Verification items for the finished model (mm, model axes). A direction names the side the tool comes from. Round coordinates to 2 decimals unless told otherwise and drop trailing zeros. Write each loop counter-clockwise with the first axis right and the second up, starting at its lowest first coordinate (ties: lowest second). Pieces come first, ordered by that corner, then holes. Notation, with made-up numbers: (20.5, -14) -> (37.5, -14) arc R17 cw to (37.5, 3) -> close; hole circle Ø11 at (21, 75.25). An arc over 180 degrees is marked (long way). Use CSV: the item, a comma, the result in double quotes.
```python
from build123d import *

# Parameters (mm, degrees)
FILLET1_R = 10


with BuildPart() as part:
    # Sketch1 → Revolve1 (revolve)
    with BuildSketch(Plane.XY, mode=Mode.PRIVATE) as revolve1_sk:
        Polygon((0, 406.66959799), (0, 416.66959799), (-100, 416.66959799), (-195, -406.33040201), (0, -406.33040201), (0, -396.33040201), (-188.812485751, -396.33040201), (-96.121112726, 406.66959799), align=None)
    revolve(revolve1_sk.sketch.rotate(Axis((0, 416.66959799, 0), (0, -1, 0)), 270), axis=Axis((0, 416.66959799, 0), (0, -1, 0)))

    # Fillet1
    fillet1_edges = [part.edges().sort_by_distance(p)[0] for p in [
        (0, 416.66959799, -100),
    ]]
    fillet(fillet1_edges, radius=FILLET1_R)


solid = part.part
```
Q1. Section check C-C (y = 112). Record the cut outline in (x, z), plus the area to 3 significant figures.
Filled in:
outline,"circle Ø270.34 at (0, 0); hole circle Ø260.27 at (0, 0)"
area,"4,200 mm²"
Q2. Section check D-D (y = -38.5). Record the cut outline in (x, z), plus the area to 3 significant figures.
Filled in:
outline,"circle Ø305.08 at (0, 0); hole circle Ø295.02 at (0, 0)"
area,"4,740 mm²"
Q3. Go/stop test with flat-tipped pins: P1, Ø1.5, axis at y = 105, z = 80.5, coming from the +X side; P2, Ø8, axis at y = 277.5, z = -52, coming from the +X side; P3, Ø3, axis at x = -97.5, z = -24, coming from the +Y side. Record where each tip stops, or that it passes through.
Filled in:
P1,"x = 110.14"
P2,"x = 105.74"
P3,"y = 412.9"
Q4. Mould release check, pull along Z, two halves, no side actions. Record for faces 1 (the flat face through (-3, -396.33, 3)), 2 (the flat face through (-1, 416.67, 1)), 3 (the conical face through (-44.656, -4.956, 141.804)): released by +Z, released by -Z, zero draft, split by the parting line, or undercut.
Filled in:
face 1,"undercut"
face 2,"zero draft"
face 3,"split by the parting line"
Q5. Section check A-A (z = 0). Record the cut outline in (x, y), plus the area to 3 significant figures.
Filled in:
outline,"(-195, -406.33) -> (195, -406.33) -> (101.02, 407.82) arc R10 ccw to (91.09, 416.67) -> (-91.09, 416.67) arc R10 ccw to (-101.02, 407.82) -> close; hole (-188.81, -396.33) -> (188.81, -396.33) -> (96.12, 406.67) -> (-96.12, 406.67) -> close"
area,"14,000 mm²"
Q6. Access from +Z, -Z, +X, -X, +Y, -Y to the whole of each face (thin tool, end or side, straight path). Record for faces 4 (the flat face through (-1, 406.67, -1)), 5 (the flat face through (-3, -406.33, -3)).
Filled in:
face 4,"none"
face 5,"+Z, -Z, +X, -X, -Y"
Q7. Section check B-B (x = 0). Record the cut outline in (y, z), plus the area to 3 significant figures.
Filled in:
outline,"(-406.33, -195) -> (407.82, -101.02) arc R10 ccw to (416.67, -91.09) -> (416.67, 91.09) arc R10 ccw to (407.82, 101.02) -> (-406.33, 195) -> close; hole (-396.33, -188.81) -> (406.67, -96.12) -> (406.67, 96.12) -> (-396.33, 188.81) -> close"
area,"14,000 mm²"
Q8. Material ranges on L1, parallel to Y at x = -20.5, z = -73; L2, parallel to X at y = 184, z = -39; L3, parallel to Z at x = 40.5, y = 27, recorded low to high.
Filled in:
L1,"-406.33 to -396.33, 406.67 to 416.67"
L2,"-120.71 to -115.41, 115.41 to 120.71"
L3,"-139.21 to -133.96, 133.96 to 139.21"
